CAD build for the part. Positions are in the model's coordinates, mm. A direction names the side the tool comes from. Round coordinates to 2 decimals unless told otherwise and drop trailing zeros. Loops run counter-clockwise (first coordinate to the right, second up) from the corner with the lowest first, then second, coordinate; pieces in that order, holes last. Notation, with made-up numbers: M 38.5,-38.75 L 58.5,-38.75 A23 cw 58.5,-27.75 Z; hole C -30,48.25 d6. An arc over 180 degrees is marked long. Use a Markdown table: item, result. Add a question column.
(1) Band-saw the part on C-C, the plane z = 8. Write the cut outline in (x, y).
(2) Wall check: L1, parallel to Y at x = 26.5, z = 25; L2, parallel to X at y = -1.5, z = 21.5; L3, parallel to Y at x = -12, z = 32.5. Give the ranges that are in metal, low to high.
(3) Flat gauge pins, fed straight in: P1, Ø3, axis at x = -26.5, z = 17.5, coming from the -Y side; P2, Ø23, axis at x = 4, y = 3, coming from the +Z side (3 decimals); P3, Ø15.5, axis at x = 0.5, z = 13, coming from the +Y side. Where does each tip first touch, or does it go through?
(4) Band-saw the part on D-D, the plane x = -40.5. Write the cut outline in (y, z) (1 decimal).
(5) Which spindle directions (+Z, -Z, +X, -X, +Y, -Y) get a long thin tool onto all of the face, cutting with end or side? Do faces 5 (the face through (-44, 6, 27.025)), 6 (the face through (0, -12.75, 31)), 7 (the face through (51, 2, 16)), 8 (the face through (0.413, 13.613, 21.727)). Say none if no direction does.
(6) Band-saw the part on A-A, the plane x = 34.5. Write the cut outline in (y, z) (3 decimals), and give its area (3 significant figures).
(7) Two-plate mould, pull along X, no slides. Class faces 1 (the face through (-50.014, 0.559, 15.389)), 2 (the face through (10, 13, 35.025)), 3 (the face through (44.39, 15.71, 0.22)), 4 (the face through (-42.445, 7.979, 20.152)): released by +X, released by -X, zero draft, split by the parting line, or undercut.
(8) Band-saw the part on B-B, the plane y = -6.5. Write the cut outline in (x, z) (3 decimals).
from build123d import *

# Parameters (mm, degrees)
BOSS_EXTRUDE12_DEPTH            = 80
CUT_EXTRUDE10_DEPTH             = 114.712356409
CUT_EXTRUDE10_DEPTH_BACK        = 114.712356409
SKETCH37_W                      = 102
SKETCH37_H                      = 56
BOSS_EXTRUDE16_DEPTH            = 3
CUT_EXTRUDE11_DEPTH             = 102.766059637
SKETCH40_W                      = 127.486838651
SKETCH40_H                      = 54.833163407
CUT_EXTRUDE12_DEPTH             = 102.007241851
CUT_EXTRUDE12_DIRECTION_2_REACH = 103.007
CUT_EXTRUDE14_DEPTH             = 18.5
F_1_4_0_25_DIAMETER_HOLE1_D     = 6.35
F_1_4_0_25_DIAMETER_HOLE1_DEPTH = 5
F_1_4_0_25_DIAMETER_HOLE1_TIP   = 1.907732465
CHAMFER2_SIZE                   = 12
CHAMFER3_SIZE                   = 2


with BuildPart() as part:
    # Sketch22 → Boss-Extrude12 (new body)
    with BuildSketch(Plane.XY):
        with BuildLine():
            Line((32.5, -14.5), (-32.5, -14.5))
            ThreePointArc((-32.5, -14.5), (-47, 0), (-32.5, 14.5))
            Line((-32.5, 14.5), (32.5, 14.5))
            ThreePointArc((32.5, 14.5), (47, 0), (32.5, -14.5))
        make_face()
    extrude(amount=BOSS_EXTRUDE12_DEPTH)

    # Sketch35 → Cut-Extrude10 (cut, two sides: drawn at the far end of the back side and taken through both)
    with BuildSketch(Plane(origin=(-32.5, 0, 0), x_dir=(0, 0, -1), z_dir=(1, 0, 0)).offset(-CUT_EXTRUDE10_DEPTH_BACK)):
        Polygon((0, 14.5), (-29.026860374, -14.5), (0, -14.5), align=None)
    extrude(amount=CUT_EXTRUDE10_DEPTH + CUT_EXTRUDE10_DEPTH_BACK, mode=Mode.SUBTRACT)

    # Sketch37 → Boss-Extrude16 (add)
    with BuildSketch(Plane(origin=(0, 7.256711984, 7.249996893), x_dir=(-1, 0, 0), z_dir=(0, -0.7074340219640284, -0.7067793888957138))):
        with Locations((0, -10.26729429)):
            Rectangle(SKETCH37_W, SKETCH37_H)
    extrude(amount=-BOSS_EXTRUDE16_DEPTH)

    # Sketch38 → Cut-Extrude11 (cut, through all)
    with BuildSketch(Plane.XY.offset(80)):
        with BuildLine():
            Line((-32.5, 12.75), (32.5, 12.75))
            ThreePointArc((32.5, 12.75), (45.25, 0), (32.5, -12.75))
            Line((32.5, -12.75), (-32.5, -12.75))
            ThreePointArc((-32.5, -12.75), (-45.25, 0), (-32.5, 12.75))
        make_face()
    extrude(amount=-CUT_EXTRUDE11_DEPTH, mode=Mode.SUBTRACT)

    # Sketch40 → Cut-Extrude12 (cut)
    with BuildSketch(Plane(origin=(0, -12.75, 0), x_dir=(1, 0, 0), z_dir=(0, 1, 0))):
        with Locations((5.984726224, -62.441589639)):
            Rectangle(SKETCH40_W, SKETCH40_H)
    extrude(amount=CUT_EXTRUDE12_DEPTH, mode=Mode.SUBTRACT)

    # Cut-Extrude12 direction 2: up to this face of the body (flat: up to its plane)
    cut_extrude12_direction_2_end = Plane(part.part.faces().sort_by_distance((0, -14.5, 56.635733163))[0])
    # Sketch40 → Cut-Extrude12 direction 2 (cut, up to the picked face)
    with BuildSketch(Plane(origin=(0, -12.75, 0), x_dir=(1, 0, 0), z_dir=(0, 1, 0)), mode=Mode.PRIVATE) as cut_extrude12_direction_2_sk1:
        with Locations((5.984726224, -62.441589639)):
            Rectangle(SKETCH40_W, SKETCH40_H)
    cut_extrude12_direction_2_tool1 = split(extrude(cut_extrude12_direction_2_sk1.sketch, amount=-CUT_EXTRUDE12_DIRECTION_2_REACH, mode=Mode.PRIVATE), bisect_by=cut_extrude12_direction_2_end, keep=Keep.BOTH, mode=Mode.PRIVATE)
    add(cut_extrude12_direction_2_tool1.solids().sort_by(Axis((5.984726, -12.75, 62.44159), (0, -1, 0)))[0], mode=Mode.SUBTRACT)

    # Sketch42 → Cut-Extrude14 (cut)
    with BuildSketch(Plane.ZY.offset(51)):
        Polygon((35.025007935, 14.5), (27.025007935, 14.5), (27.025007935, -8.259321849), (33.271466325, -14.5), (35.025007935, -14.5), align=None)
    extrude(amount=-CUT_EXTRUDE14_DEPTH, mode=Mode.SUBTRACT)

    # 1/4 (0.25) Diameter Hole1
    with Locations(Plane(origin=(0, 14.5, 0), x_dir=(1, 0, 0), z_dir=(0, 1, 0))):
        with Locations((2.6293e-05, -24.875007935)):
            Hole(F_1_4_0_25_DIAMETER_HOLE1_D / 2, depth=F_1_4_0_25_DIAMETER_HOLE1_DEPTH)
            with Locations((0, 0, -(F_1_4_0_25_DIAMETER_HOLE1_DEPTH + F_1_4_0_25_DIAMETER_HOLE1_TIP / 2))):  # 118° drill point
                Cone(0, F_1_4_0_25_DIAMETER_HOLE1_D / 2, F_1_4_0_25_DIAMETER_HOLE1_TIP, mode=Mode.SUBTRACT)

    # Chamfer2
    chamfer2_edges = [part.edges().sort_by_distance(p)[0] for p in [
        (51, -18.728671856, 35.381751886),
        (51, 20.850973922, -4.234553344),
        (-51, 20.850973922, -4.234553344),
        (-51, -18.728671856, 35.381751886),
    ]]
    chamfer(chamfer2_edges, length=CHAMFER2_SIZE)

    # Chamfer3
    chamfer3_edges = [part.edges().sort_by_distance(p)[0] for p in [
        (-51, 0, 14.513430187),
        (51, 0, 14.513430187),
        (0, -19.789822889, 34.321582802),
        (0, 19.789822889, -5.294722428),
        (-45, -15.549146556, 30.07697867),
        (45, -15.549146556, 30.07697867),
        (45, 15.549146556, -1.050118296),
        (-45, 15.549146556, -1.050118296),
    ]]
    chamfer(chamfer3_edges, length=CHAMFER3_SIZE)


solid = part.part
Return value:
| question | item | result |
|---|---|---|
| 1 | outline | M -51,9.33 L -49,6.51 L -43.46,6.51 A12.75 cw -32.5,12.75 L 32.5,12.75 A12.75 cw 43.46,6.51 L 49,6.51 L 51,9.33 L 51,10.75 L 42.23,10.75 A14.5 ccw 32.5,14.5 L -32.5,14.5 A14.5 ccw -42.23,10.75 L -51,10.75 Z |
| 2 | L1 | 12.75 to 14.5 |
| 2 | L2 | -46.92 to -45.16, 45.16 to 46.92 |
| 2 | L3 | -17.97 to -12.75, 12.75 to 14.5 |
| 3 | P1 | y = 12.75 |
| 3 | P2 | z = 35.025 |
| 3 | P3 | y = 14.5 |
| 4 | outline | M -17.3,34.7 L -16.7,31.3 L -9.9,24.5 L -9.9,28.7 L -16.6,35.4 Z; M 9.9,4.6 L 16.7,-2.2 L 20.1,-2.8 L 20.9,-2.1 L 12.1,6.7 L 12.1,27 L 9.9,27 Z |
| 5 | face 5 | +Z, -X, +Y |
| 5 | face 6 | +Z, -Z |
| 5 | face 7 | +Z, -Z, +X, +Y, -Y |
| 5 | face 8 | +Y |
| 6 | outline | M -18.376,32.907 L -12.592,27.117 L -12.592,35.025 L -14.361,35.025 L -14.361,33.133 L -17.668,36.442 L -18.375,35.735 Z; M 12.592,1.91 L 18.376,-3.88 L 21.205,-3.881 L 21.912,-3.174 L 14.361,4.383 L 14.361,35.025 L 12.592,35.025 Z |
| 6 | area | 115 mm^2 |
| 7 | face 1 | released by -X |
| 7 | face 2 | zero draft |
| 7 | face 3 | released by +X |
| 7 | face 4 | undercut |
| 8 | outline | M -51,23.849 L -49,21.019 L -43.469,21.019 L -43.469,27.025 L -45.461,27.025 L -45.461,25.264 L -51,25.264 Z; M 43.469,21.019 L 49,21.019 L 51,23.849 L 51,25.264 L 45.461,25.264 L 45.461,35.025 L 43.469,35.025 Z |
